Model file for the job. Use its own axes, mm. A direction names the side the tool comes from. Round coordinates to 2 decimals unless told otherwise and drop trailing zeros. Order: outer loops, then holes, each group sorted by start corner. A loop starts at its lowest first (then second) coordinate and runs counter-clockwise, first axis right, second up. Notation, with made-up numbers: (9, -6.75) - (43, -6.75) arc R21 ccw to (43, 28.25) - close; hole circle Ø1 at (72.25, 64.5). An arc over 180 degrees is marked (long way). Use one line per item in the form item = value.
from build123d import *

# Parameters (mm, degrees)
BOSS_EXTRUDE1_DEPTH      = 50
BOSS_EXTRUDE1_DEPTH_BACK = 10
SKETCH2_R                = 8
SKETCH4_R                = 4.21
CUT_EXTRUDE3_DEPTH       = 50


with BuildPart() as part:
    # Sketch1 → Revolve1 (revolve)
    with BuildSketch(Plane(origin=(0, 0, 0), x_dir=(1, 0, 0), z_dir=(0, 1, 0))):
        with BuildLine():
            Line((0, 30), (0, -30))
            ThreePointArc((0, -30), (30, 0), (0, 30))
        make_face()
    revolve(axis=Axis((0, 0, -30), (0, 0, 1)))

    # Sketch2 → Boss-Extrude1 (add, two sides: drawn at the far end of the back side and taken through both)
    with BuildSketch(Plane(origin=(0, 30, 0), x_dir=(1, 0, 0), z_dir=(0, 1, 0)).offset(-BOSS_EXTRUDE1_DEPTH_BACK)):
        with Locations(Location((0, 0, 0), (0, 0, 270))):
            Circle(SKETCH2_R)
    extrude(amount=BOSS_EXTRUDE1_DEPTH + BOSS_EXTRUDE1_DEPTH_BACK)

    # Sketch4 → Cut-Extrude3 (cut)
    with BuildSketch(Plane(origin=(0, 80, 0), x_dir=(1, 0, 0), z_dir=(0, 1, 0))):
        with Locations(Location((0, 0, 0), (0, 0, 270))):
            Circle(SKETCH4_R)
    extrude(amount=-CUT_EXTRUDE3_DEPTH, mode=Mode.SUBTRACT)


solid = part.part
(1) Slice it at A-A on z = 0. Give the cut face in (x, y), then the cut area to 3 significant figures.
Report:
outline = (-8, 28.91) arc R30 ccw (long way) to (8, 28.91) - (8, 80) - (4.21, 80) - (4.21, 30) - (-4.21, 30) - (-4.21, 80) - (-8, 80) - close
area = 3,210 mm2
(2) Probe probe 1 along X at (y, z) = (44, 0); probe 2 along Z at (x, y) = (-2, 14); probe 3 along X at (y, z) = (66.5, -6). List the from-to ranges inside material, lowest first. Write a range as [from, to].
Report:
probe_1 = [-8, -4.21], [4.21, 8]
probe_2 = [-26.46, 26.46]
probe_3 = [-5.29, 5.29]
(3) Slice it at C-C on y = 48.5. Give the cut face in (x, z).
Report:
outline = circle Ø16 at (0, 0); hole circle Ø8.42 at (0, 0)
(4) Slice it at D-D on y = -22. Give the cut face in (x, z), then the cut area to 3 significant figures.
Report:
outline = circle Ø40.79 at (0, 0)
area = 1,310 mm2
(5) Slice it at B-B on x = 0. Give the cut face in (y, z).
Report:
outline = (28.91, -8) - (80, -8) - (80, -4.21) - (30, -4.21) - (30, 4.21) - (80, 4.21) - (80, 8) - (28.91, 8) arc R30 ccw (long way) to start
(6) Pin check, flat tips, straight feed: pin 1 (1.5 mm diameter, centred on y = -9, z = 2.5, fed in from +X); pin 2 (2 mm diameter, centred on x = 14.5, z = -10, fed in from +Y); pin 3 (1.5 mm diameter, centred on x = -8.5, z = -11.5, fed in from -Y). Stop position of each tip, or through.
Report:
pin_1 = 28.74
pin_2 = 24.98
pin_3 = -26.77
(7) Tool access for faces 1 (the face through (-3.4, 80, 3.4)), 2 (the face through (1.265, 55.35, 4.016)): list every direction of +Z, -Z, +X, -X, +Y, -Y with a clear straight run to the whole face (end or side of a thin tool).
Report:
face_1 = +Z, -Z, +X, -X, +Y
face_2 = +Y
